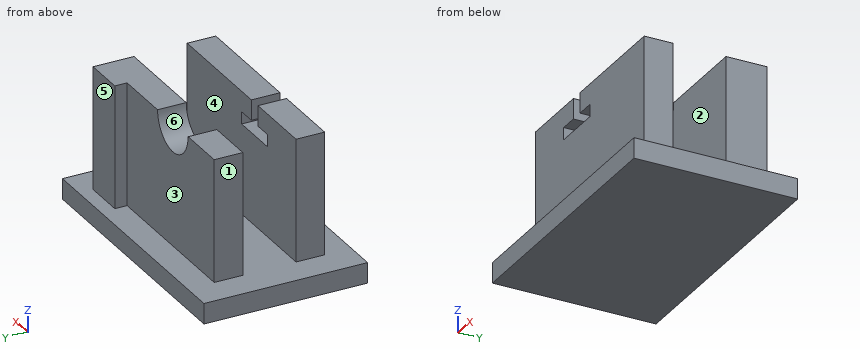
from build123d import *

# Parameters (mm, degrees)
SKETCH_1_W          = 65
SKETCH_1_H          = 40
EXTRUDE_1_DEPTH     = 5
SKETCH_2_W          = 50
SKETCH_2_H          = 7
SKETCH_2_W_2        = 10
SKETCH_2_H_2        = 3
EXTRUDE_2_DEPTH     = 30
SKETCH_4_R          = 7
CUT_EXTRUDE_1_DEPTH = 7
SKETCH_7_W          = 12
SKETCH_7_H          = 3
SKETCH_7_W_2        = 3
SKETCH_7_H_2        = 5
CUT_EXTRUDE_3_DEPTH = 7


with BuildPart() as part:
    # Эскиз1 → Бобышка-Вытянуть1 (new body)
    with BuildSketch(Plane.XY):
        Rectangle(SKETCH_1_W, SKETCH_1_H)
    extrude(amount=EXTRUDE_1_DEPTH)

    # Эскиз2 → Бобышка-Вытянуть2 (add)
    with BuildSketch(Plane.XY.offset(5)):
        with Locations((0, 10)):
            Rectangle(SKETCH_2_W, SKETCH_2_H)
        with Locations((20, 15)):
            Rectangle(SKETCH_2_W_2, SKETCH_2_H_2)
        with Locations((0, -10)):
            Rectangle(SKETCH_2_W, SKETCH_2_H)
    extrude(amount=EXTRUDE_2_DEPTH)

    # Эскиз4 → Вырез-Вытянуть1 (cut)
    with BuildSketch(Plane(origin=(0, 13.5, 0), x_dir=(1, 0, 0), z_dir=(0, 1, 0))):
        with Locations((-6, -35)):
            Circle(SKETCH_4_R)
    extrude(amount=-CUT_EXTRUDE_1_DEPTH, mode=Mode.SUBTRACT)

    # Эскиз7 → Вырез-Вытянуть3 (cut)
    with BuildSketch(Plane.XZ.offset(13.5)):
        with Locations((-6, 28.5)):
            Rectangle(SKETCH_7_W, SKETCH_7_H)
        with Locations((-6, 32.5)):
            Rectangle(SKETCH_7_W_2, SKETCH_7_H_2)
    extrude(amount=-CUT_EXTRUDE_3_DEPTH, mode=Mode.SUBTRACT)


solid = part.part
Model file for the job. Use its own axes, mm. Face numbers are marked on the shaded views. A direction names the side the tool comes from. Round coordinates to 2 decimals unless told otherwise and drop trailing zeros. Order: outer loops, then holes, each group sorted by start corner. A loop starts at its lowest first (then second) coordinate and runs counter-clockwise, first axis right, second up. Notation, with made-up numbers: M 44,-30.5 L 73,-30.5 A25 ccw 73,-3.5 Z; hole C 7.5,55.5 d10. An arc over 180 degrees is marked long. Write each question's results on one line, items separated by ' | '. Start each with the question number.
(1) Which spindle directions (+Z, -Z, +X, -X, +Y, -Y) get a long thin tool onto all of the face, cutting with end or side? Do the marked faces 1, 2 and 3. Say none if no direction does.
(2) Saw through at C-C, the plane z = 31. Give the cut face in (x, y), then the cut area to 3 significant figures.
(3) Saw through at D-D, the plane y = 3.5. Give the cut face in (x, z), then the cut area to 3 significant figures.
(4) Two-plate mould, pull along Y, no slides. Class the marked faces 4, 5 and 6: pulls with the +Y half, pulls with the -Y half, needs draft (parallel to the pull), parting line crosses it, or undercut.
(5) Saw through at A-A, the plane z = 25. Give the cut face in (x, y).
(6) Probe probe 1 along Y at (x, z) = (8, 7); probe 2 along Y at (x, z) = (22.5, 6.5); probe 3 along X at (y, z) = (-7, 28). List the from-to ranges inside material, lowest first. Write a range as from..to.
(7) Drop flat-ended pins along their axis: pin 1 (4 mm diameter, centred on y = -11.5, z = 31.5, fed in from -X); pin 2 (1 mm diameter, centred on x = -5.5, y = -8.5, fed in from +Z); pin 3 (8 mm diameter, centred on y = 12, z = 21, fed in from +X). Give the stop position or say it passes through.
(8) Saw through at B-B, the plane x = -6. Give the cut face in (y, z).
Established:
1) face 1: +Z, -X, +Y, -Y | face 2: +Z, +X, -X | face 3: +Z, -X, +Y
2) outline: M -25,-13.5 L -7.5,-13.5 L -7.5,-6.5 L -25,-6.5 Z; M -25,6.5 L -11.74,6.5 L -11.74,13.5 L -25,13.5 Z; M -4.5,-13.5 L 25,-13.5 L 25,-6.5 L -4.5,-6.5 Z; M -0.26,6.5 L 25,6.5 L 25,16.5 L 15,16.5 L 15,13.5 L -0.26,13.5 Z | area: 629 mm^2
3) outline: M -32.5,0 L 32.5,0 L 32.5,5 L -32.5,5 Z | area: 325 mm^2
4) face 4: undercut | face 5: pulls with the +Y half | face 6: needs draft
5) outline: M -25,-13.5 L 25,-13.5 L 25,-6.5 L -25,-6.5 Z; M -25,6.5 L 25,6.5 L 25,16.5 L 15,16.5 L 15,13.5 L -25,13.5 Z
6) probe 1: y = -13.5..-6.5, 6.5..13.5 | probe 2: y = -13.5..-6.5, 6.5..16.5 | probe 3: x = -25..-12, 0..25
7) pin 1: stops at x = -25 | pin 2: stops at z = 27 | pin 3: stops at x = 25
8) outline: M -20,0 L 20,0 L 20,5 L 13.5,5 L 13.5,28 L 6.5,28 L 6.5,5 L -6.5,5 L -6.5,27 L -13.5,27 L -13.5,5 L -20,5 Z
